Read the model definition and answer for the solid it produces. Units are mm, in the model's axes. Round coordinates to 2 decimals unless told otherwise and drop trailing zeros. Order: outer loops, then holes, each group sorted by start corner. A loop starts at its lowest first (then second) coordinate and runs counter-clockwise, first axis right, second up. Notation, with made-up numbers: (84, -28.75) - (107, -28.75) arc R14 ccw to (107, -13.75) - close; hole circle Ø4 at (-8.5, 30.25). An arc over 180 degrees is marked (long way). Answer as a JSON object with one key per item and string values. Group by question number.
Q1. Given pin 1 Ø3 at (x, z) = (11.5, 3) entering from -Y; pin 2 Ø5 at (x, z) = (15, -3.5) entering from +Y; pin 3 Ø3 at (x, z) = (-0.5, -3) entering from -Y, each flat-ended and moving along its own axis, determine where each tip first touches the part or whether it passes through.
Q2. A cutting plane is placed at A-A on x = 4. Determine the outline of the cut face in (y, z), and give its area (3 significant figures).
Q3. Consider line 1 (X direction, y = -3.25, z = -2.25); line 2 (Z direction, x = 13, y = 0); line 3 (X direction, y = 3.75, z = -2.75). Determine where each line is inside the solid, lowest interval first.
Autodesk Inventor part; units mm, degrees
ref_plane "YZ Plane" through (0, 0, 0) normal (1, 0, 0) x (0, 1, 0)
ref_plane "XZ Plane" through (0, 0, 0) normal (0, 1, 0) x (-1, 0, 0)
ref_plane "XY Plane" through (0, 0, 0) normal (0, 0, 1) x (1, 0, 0)
sketch "Sketch1" plane through (0, 0, 0) normal (0, 0, 1) x (1, 0, 0)
  line L0 (0, 0) -> (15, 0)
  line L1 (15, 0) -> (15, 3.75)
  line L2 (15, 3.75) -> (0, 3.75)
  line L3 (0, 3.75) -> (0, 0)
  line L4 (0, 3.75) -> (0, 5.1962)
  line L5 (15, 3.75) -> (15, 5.1962)
  arc A0 (18, 0) -> (15, 5.1962) centre (12, 0) ccw
  arc A1 (0, 5.1962) -> (-3, 0) centre (3, 0) ccw
  line L6 (0, 0) -> (-3, 0)
  line L7 (15, 0) -> (18, 0)
  dimension "d0" = 15
  dimension "d1" = 3.75
  dimension "d2" = 6
  dimension "d3" = 6
  dimension "d4" = 3
  dimension "d5" = 3
revolve "Revolution1" add sketch "Sketch1" angle 360 about axis through (0, 0, 0) along (1, 0, 0)
chamfer "Chamfer1" distance 0.5 angle 45 2 edges at (0, -5.1962, 0) (15, -5.1962, 0)
properties part number "Claw Axis(1)" material "Stainless Steel"
Result set:
{
 "1": {"pin 1": "stops at y = -3.44", "pin 2": "stops at y = 4.82", "pin 3": "stops at y = -4.69"},
 "2": {"outline": "circle Ø7.5 at (0, 0)", "area": "44.2 mm²"},
 "3": {"line 1": "x = -1.51 to 0, 15 to 16.51", "line 2": "z = -3.75 to 3.75", "line 3": "x = -0.79 to 0, 15 to 15.79"}
}
